Build history of the part. All positions in model axes, mm. A direction names the side the tool comes from. Round coordinates to 2 decimals unless told otherwise and drop trailing zeros. Write each loop counter-clockwise with the first axis right and the second up, starting at its lowest first coordinate (ties: lowest second). Pieces come first, ordered by that corner, then holes. Notation, with made-up numbers: M -6.75,85.25 L 40.25,85.25 A6 cw 40.25,93.25 Z; hole C 76.25,24.25 d5. An arc over 180 degrees is marked long. Write item = value, one per line.
from build123d import *

# Parameters (mm, degrees)
BOSS_EXTRUDE1_DEPTH = 50
SKETCH4_R           = 16.890804547
BOSS_EXTRUDE2_DEPTH = 62.458045


with BuildPart() as part:
    # Sketch2 → Boss-Extrude1 (new, symmetric)
    with BuildSketch(Plane(origin=(0, 0, 0), x_dir=(0, 0, -1), z_dir=(1, 0, 0))):
        Polygon((0, 0), (59.188081664, 0), (59.188081664, 110.495775099), (0, 110.495775099), (0, 98.172971619), (45.177222912, 98.172971619), (45.177222912, 78.929141526), (0, 78.929141526), (0, 65.255893829), (45.177222912, 65.255893829), (45.177222912, 48.037730062), (0, 48.037730062), (0, 34.195676837), (45.177222912, 34.195676837), (45.177222912, 17.652735178), (0, 17.652735178), align=None)
    extrude(amount=BOSS_EXTRUDE1_DEPTH, both=True)

    # Sketch4 → Boss-Extrude2 (add)
    with BuildSketch(Plane(origin=(0, 110.495775099, 0), x_dir=(1, 0, 0), z_dir=(0, 1, 0))):
        with Locations((0, 32.021799432)):
            Circle(SKETCH4_R)
    extrude(amount=-BOSS_EXTRUDE2_DEPTH)


solid = part.part
1. Probe probe 1 along Y at (x, z) = (34.5, -36); probe 2 along Y at (x, z) = (10, -19.5); probe 3 along Z at (x, y) = (-36.5, 18). List the from-to ranges inside material, lowest first.
Responses:
probe_1 = 0 to 17.65, 34.2 to 48.04, 65.26 to 78.93, 98.17 to 110.5
probe_2 = 0 to 17.65, 34.2 to 110.5
probe_3 = -59.19 to -45.18
2. Band-saw the part on C-C (y = 92.5). List the corners of the cut face in (x, z), plus the area to 3 significant figures.
Responses:
outline = M -50,-59.19 L 50,-59.19 L 50,-45.18 L 10.59,-45.18 A16.89 ccw long -10.59,-45.18 L -50,-45.18 Z
area = 2,240 mm²
3. Mould opens along Y. For faces 1 (the face through (-1, 110.496, -30)), 2 (the face through (1, 9, 0)), 3 (the face through (1, 78.929, -13)) say: pulls with the +Y half, pulls with the -Y half, needs draft (parallel to the pull), parting line crosses it, or undercut.
Responses:
face_1 = pulls with the +Y half
face_2 = needs draft
face_3 = undercut
4. Tool access for faces 4 (the face through (-0.58, 56.77, -15.14)), 5 (the face through (-30, 89, -45.177)), 6 (the face through (1, 41, 0)), 7 (the face through (1, 17.653, -23)): list every direction of +Z, -Z, +X, -X, +Y, -Y with a clear straight run to the whole face (end or side of a thin tool).
Responses:
face_4 = none
face_5 = -X
face_6 = +Z, +X, -X, +Y, -Y
face_7 = +Z, +X, -X
5. Band-saw the part on D-D (x = 0). List the corners of the cut face in (y, z), plus the area to 3 significant figures.
Responses:
outline = M 0,-59.19 L 110.5,-59.19 L 110.5,0 L 98.17,0 L 98.17,-15.13 L 78.93,-15.13 L 78.93,0 L 65.26,0 L 65.26,-15.13 L 48.04,-15.13 L 48.04,0 L 34.2,0 L 34.2,-45.18 L 17.65,-45.18 L 17.65,0 L 0,0 Z
area = 5,240 mm²
6. Flat gauge pins, fed straight in: pin 1 (9.5 mm diameter, centred on x = 29, y = 86, fed in from +Z); pin 2 (5 mm diameter, centred on y = 61, z = -24.5, fed in from +X); pin 3 (2 mm diameter, centred on y = 94, z = -29.5, fed in from +X); pin 4 (3 mm diameter, centred on y = 62.5, z = -6, fed in from +X). Where does each tip first touch, or does it go through?
Responses:
pin_1 = -45.18
pin_2 = 16.13
pin_3 = 16.82
pin_4 = through
7. Band-saw the part on B-B (x = -31.5). List the corners of the cut face in (y, z).
Responses:
outline = M 0,-59.19 L 110.5,-59.19 L 110.5,0 L 98.17,0 L 98.17,-45.18 L 78.93,-45.18 L 78.93,0 L 65.26,0 L 65.26,-45.18 L 48.04,-45.18 L 48.04,0 L 34.2,0 L 34.2,-45.18 L 17.65,-45.18 L 17.65,0 L 0,0 Z
8. Band-saw the part on A-A (z = -20). List the corners of the cut face in (x, y), plus the area to 3 significant figures.
Responses:
outline = M -50,0 L 50,0 L 50,17.65 L -50,17.65 Z; M -50,34.2 L 50,34.2 L 50,48.04 L 11.86,48.04 L 11.86,65.26 L 50,65.26 L 50,78.93 L 11.86,78.93 L 11.86,98.17 L 50,98.17 L 50,110.5 L -50,110.5 L -50,98.17 L -11.86,98.17 L -11.86,78.93 L -50,78.93 L -50,65.26 L -11.86,65.26 L -11.86,48.04 L -50,48.04 Z
area = 6,610 mm²
